```python
from build123d import *

# Parameters (mm, degrees)
SKETCH_1_W          = 285
SKETCH_1_H          = 185
EXTRUDE_1_DEPTH     = 14
SKETCH_2_R          = 2
CUT_EXTRUDE_1_DEPTH = 8
SKETCH_3_W          = 275
SKETCH_3_H          = 156
EXTRUDE_2_DEPTH     = 1


with BuildPart() as part:
    # 草图1 → 凸台-拉伸1 (new body)
    with BuildSketch(Plane(origin=(0, 0, 0), x_dir=(1, 0, 0), z_dir=(0, 1, 0))):
        Rectangle(SKETCH_1_W, SKETCH_1_H)
    extrude(amount=EXTRUDE_1_DEPTH)

    # 草图2 → 切除-拉伸1 (cut)
    with BuildSketch(Plane(origin=(0, 14, 0), x_dir=(1, 0, 0), z_dir=(0, 1, 0))):
        with Locations((-37.5, 37.5)):
            Circle(SKETCH_2_R)
        with Locations((37.5, 37.5)):
            Circle(SKETCH_2_R)
        with Locations((37.5, -37.5)):
            Circle(SKETCH_2_R)
        with Locations((-37.5, -37.5)):
            Circle(SKETCH_2_R)
    extrude(amount=-CUT_EXTRUDE_1_DEPTH, mode=Mode.SUBTRACT)

    # 草图3 → 凸台-拉伸2 (add)
    with BuildSketch(Plane.XZ):
        Polygon((-142.5, -92.5), (142.5, -92.5), (142.5, -68.5), (142.5, 92.5), (137.5, 92.5), (-137.5, 92.5), (-142.5, 92.5), (-142.5, -68.5), align=None)
        with Locations((0, 9.5)):
            Rectangle(SKETCH_3_W, SKETCH_3_H, mode=Mode.SUBTRACT)
    extrude(amount=EXTRUDE_2_DEPTH)


solid = part.part
```
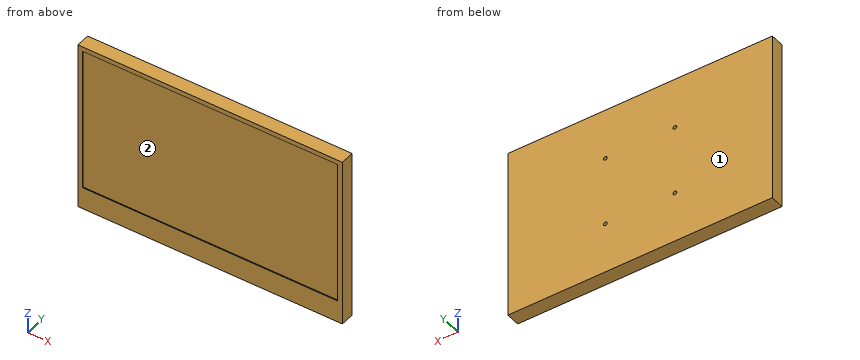
CAD build for the part. Positions are in the model's coordinates, mm. Face numbers are marked on the shaded views. Give positions to 0.01 mm unless a question says otherwise; leave off trailing zeros. Order: outer loops, then holes, each group sorted by start corner. A loop starts at its lowest first (then second) coordinate and runs counter-clockwise, first axis right, second up.
(1) Saw through at B-B, the plane x = -27. Give the cut face in (y, z), then the cut area to 3 significant figures.
(2) Flat gauge pins, fed straight in: pin 1 (2 mm diameter, centred on x = -79.5, z = -21.5, fed in from -Y); pin 2 (2 mm diameter, centred on x = -38, z = 37.5, fed in from +Y). Where does each tip first touch, or does it go through?
(3) Saw through at A-A, the plane z = 27.5. Give the cut face in (x, y).
(4) Drill centre lines: L1, parallel to X at y = 9.5, z = -37.5; L2, parallel to Z at x = -37.5, y = 11.5; L3, parallel to Y at x = 72.5, z = 74.5. Where is each one in solid material? Low to high.
(5) Mould opens along Z. For the marked faces 1 and 2 say: released by +Z, released by -Z, zero draft, split by the parting line, or undercut.
Results found:
1. outline: (-1, -92.5) - (14, -92.5) - (14, 92.5) - (-1, 92.5) - (-1, 87.5) - (0, 87.5) - (0, -68.5) - (-1, -68.5) - close
1. area: 2,620 mm2
2. pin 1: stops at y = 0
2. pin 2: stops at y = 6
3. outline: (-142.5, -1) - (-137.5, -1) - (-137.5, 0) - (137.5, 0) - (137.5, -1) - (142.5, -1) - (142.5, 14) - (-142.5, 14) - close
4. L1: x = -142.5 to -39.5, -35.5 to 35.5, 39.5 to 142.5
4. L2: z = -92.5 to -39.5, -35.5 to 35.5, 39.5 to 92.5
4. L3: y = 0 to 14
5. face 1: zero draft
5. face 2: undercut
